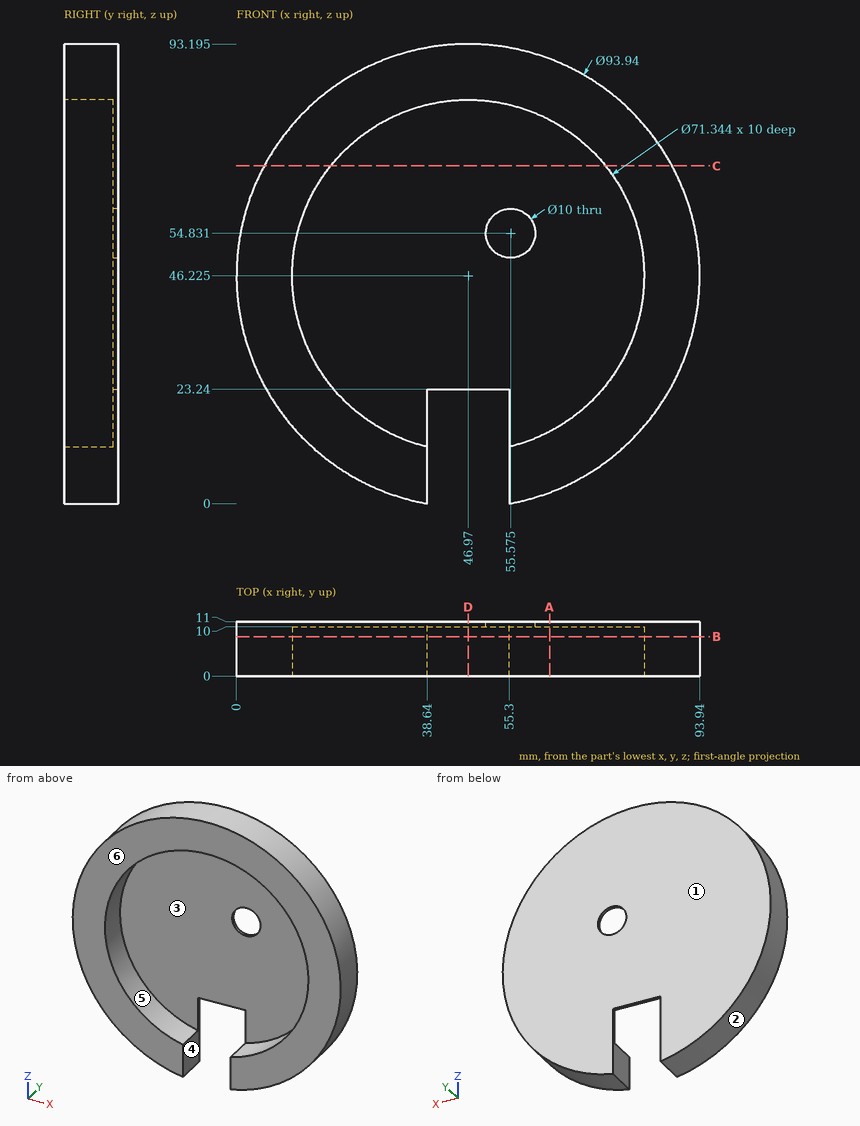
For this review, use the dimensioned drawing (mm, ordinates from the lowest corner) and the shaded views. A direction names the side the tool comes from. Give positions to 0.01 mm unless a question says otherwise; leave off trailing zeros. Loops run counter-clockwise (first coordinate to the right, second up) from the corner with the lowest first, then second, coordinate; pieces in that order, holes last.
Item 1: Take a section at C-C, the plane z = 68.5. State the section outline as (x, y) points.
Item 2: For line 1 along X through (y, z) = (8.5, 45) (1 decimal); line 2 along Z through (x, y) = (46.97, 4.5) (1 decimal); line 3 along X through (y, z) = (2.5, 51.5), list the stretches that pass through material, from the lowest coordinate up.
Item 3: Take a section at A-A, the plane x = 63.5. State the section outline as (y, z) points (1 decimal).
Item 4: Draft analysis for pull direction Z (two halves, no side actions). For the marked faces 1, 2 and 3, state which applies: +Z half, -Z half, draft (parallel to the pull), parting line (faces both ways), or undercut.
Item 5: Insertion check: pin 1 (1.1 mm diameter, centred on x = 44.5, y = 10.5, fed in from -Z); pin 2 (6 mm diameter, centred on y = 5, z = 77, fed in from +X); pin 3 (3 mm diameter, centred on x = 75.5, z = 50.5, fed in from -Y); pin 4 (11.5 mm diameter, centred on x = 55.58, z = 54.83, fed in from +Y). Each pin has a flat end and moves straight along its axis. Give the tip position at first contact, or say it passes through.
Item 6: Tool access review of the marked faces 4, 5 and 6: name each direction out of +Z, -Z, +X, -X, +Y, -Y from which nothing blocks a thin tool from reaching the whole face with its end or side.
Item 7: Take a section at D-D, the plane x = 46.97. State the section outline as (y, z) points (1 decimal).
Item 8: Take a section at B-B, the plane y = 8. State the section outline as (x, z) points (1 decimal).
Calculated:
1. outline: (5.62, 0) - (19.11, 0) - (19.11, 10) - (74.83, 10) - (74.83, 0) - (88.32, 0) - (88.32, 11) - (5.62, 11) - close
2. line 1: x = 0 to 11.3, 82.6 to 93.9
2. line 2: z = 81.9 to 93.2
2. line 3: x = 0.3 to 11.69, 82.25 to 93.64
3. outline: (0, 2.3) - (11, 2.3) - (11, 90.2) - (0, 90.2) - (0, 77.8) - (10, 77.8) - (10, 14.6) - (0, 14.6) - close
4. face 1: draft
4. face 2: parting line
4. face 3: undercut
5. pin 1: stops at z = 23.24
5. pin 2: stops at x = 84.85
5. pin 3: stops at y = 10
5. pin 4: stops at y = 11
6. face 4: -Z, +Y, -Y
6. face 5: -Y
6. face 6: +Z, -Z, +X, -X, -Y
7. outline: (0, 81.9) - (10, 81.9) - (10, 23.2) - (11, 23.2) - (11, 93.2) - (0, 93.2) - close
8. outline: (38.6, 0) - (38.6, 11.5) arc R35.7 cw (long way) to (55.3, 11.5) - (55.3, 0) arc R47 ccw (long way) to start
